```python
from build123d import *

# Parameters (mm, degrees)
BOSS_EXTRUDE1_DEPTH = 700
SKETCH3_W           = 125
SKETCH3_H           = 60
CUT_EXTRUDE1_DEPTH  = 706.00443261
CHAMFER1_SIZE       = 30
SKETCH4_R           = 10
CUT_EXTRUDE2_DEPTH  = 708.990112925
SKETCH5_R           = 7.5
CUT_EXTRUDE3_DEPTH  = 708.990112925
CHAMFER2_SIZE       = 3
FILLET1_R           = 3


with BuildPart() as part:
    # Sketch1 → Boss-Extrude1 (new body)
    with BuildSketch(Plane.XY):
        Polygon((0, -37.5), (0, 37.5), (75, 37.5), (75, 31.15), (6.35, 31.15), (6.35, -31.15), (75, -31.15), (75, -37.5), align=None)
    extrude(amount=BOSS_EXTRUDE1_DEPTH)

    # Sketch3 → Cut-Extrude1 (cut, through all)
    with BuildSketch(Plane.ZY):
        with Locations((92.5, 0)):
            Rectangle(SKETCH3_W, SKETCH3_H)
        with Locations((607.5, 0)):
            Rectangle(SKETCH3_W, SKETCH3_H)
        Polygon((400, 10.383333333), (373, 10.383333333), (373, 31.15), (327, 31.15), (307, 31.15), (307, 10.383333333), (300, 10.383333333), (270, 10.383333333), (270, -10.383333333), (300, -10.383333333), (327, -10.383333333), (327, -31.15), (373, -31.15), (393, -31.15), (393, -10.383333333), (400, -10.383333333), align=None)
    extrude(amount=-CUT_EXTRUDE1_DEPTH, mode=Mode.SUBTRACT)

    # Chamfer1
    chamfer1_edges = [part.edges().sort_by_distance(p)[0] for p in [
        (75, -34.325, 0),
        (75, 34.325, 700),
        (75, -34.325, 700),
        (75, 34.325, 0),
    ]]
    chamfer(chamfer1_edges, length=CHAMFER1_SIZE)

    # Sketch4 → Cut-Extrude2 (cut, through all)
    with BuildSketch(Plane(origin=(0, 37.5, 0), x_dir=(1, 0, 0), z_dir=(0, 1, 0))):
        with Locations(Location((37.5, -607.5, 0), (0, 0, 270))):
            Circle(SKETCH4_R)
        with Locations(Location((37.5, -92.5, 0), (0, 0, 270))):
            Circle(SKETCH4_R)
    extrude(amount=-CUT_EXTRUDE2_DEPTH, mode=Mode.SUBTRACT)

    # Sketch5 → Cut-Extrude3 (cut, through all)
    with BuildSketch(Plane.XZ.offset(37.5)):
        with Locations(Location((38, 273.823015652, 0), (0, 0, 270))):
            Circle(SKETCH5_R)
        with Locations(Location((13.565044391, 350, 0), (0, 0, 270))):
            Circle(SKETCH5_R)
    extrude(amount=-CUT_EXTRUDE3_DEPTH, mode=Mode.SUBTRACT)

    # Chamfer2
    chamfer2_edges = [part.edges().sort_by_distance(p)[0] for p in [
        (6.35, -20.766666667, 327),
        (6.35, 0, 270),
        (6.35, 20.766666667, 373),
        (0, -20.766666667, 393),
        (0, 20.766666667, 307),
    ]]
    chamfer(chamfer2_edges, length=CHAMFER2_SIZE)

    # Fillet1
    fillet1_edges = [part.edges().sort_by_distance(p)[0] for p in [
        (1.675, 10.383333333, 270),
        (1.675, -10.383333333, 270),
        (1.675, 31.15, 373),
        (1.675, -31.15, 327),
        (4.675, -31.15, 393),
        (4.675, 31.15, 307),
        (3.175, 10.383333333, 400),
        (3.175, -10.383333333, 400),
    ]]
    fillet(fillet1_edges, radius=FILLET1_R)


solid = part.part
```
Model file for the job. Use its own axes, mm. A direction names the side the tool comes from. Coordinates: 2 decimals unless noted, no trailing zeros. Order: outer loops, then holes, each group sorted by start corner. A loop starts at its lowest first (then second) coordinate and runs counter-clockwise, first axis right, second up. Notation, with made-up numbers: (-20, 0) - (27, 0) arc R27 ccw to (27, 27) - close; hole circle Ø6 at (86.5, 1). An arc over 180 degrees is marked (long way). Return JSON: item names as keys, results as strings. Group by question number.
1) Saw through at D-D, the plane z = 364. Write the cut outline in (x, y).
2) Tool access for faces 1 (the flat face through (0, -34, 345)), 2 (the flat face through (6.35, 0, 500)): list every direction of +Z, -Z, +X, -X, +Y, -Y with a clear straight run to the whole face (end or side of a thin tool).
3) Saw through at B-B, the plane x = 57.5. Write the cut outline in (y, z).
4) Saw through at A-A, the plane z = 92.5. Write the cut outline in (x, y), plus the area to 3 significant figures.
5) Probe line 1 (Y direction, x = 41.5, z = 585.5); line 2 (X direction, y = -36, z = 92); line 3 (X direction, y = 33, z = 350). List the from-to ranges inside material, lowest first. Write a range as from..to.
6) Flat gauge pin, fed straight in: P1, Ø9, axis at x = 13.57, z = 350, coming from the -Y side. Where does the tip first touch, or does it go through?
7) Mould opens along Z. For faces 3 (the flat face through (60, 34, 685)), 4 (the flat face through (60, 34, 15)), 5 (the cylindrical face through (33.67, -34.281, 616.737)) say: released by +Z, released by -Z, zero draft, split by the parting line, or undercut.
8) Saw through at C-C, the plane y = -1.5. Write the cut outline in (x, z), plus the area to 3 significant figures.
Values found:
{
 "1": {"outline": "(0, -37.5) - (75, -37.5) - (75, -31.15) - (0, -31.15) - close; (0, 31.15) - (75, 31.15) - (75, 37.5) - (0, 37.5) - close"},
 "2": {"face 1": "+Z, -Z, -X, +Y, -Y", "face 2": "+Z, -Z, +X"},
 "3": {"outline": "(-37.5, 12.5) - (-31.15, 12.5) - (-31.15, 687.5) - (-37.5, 687.5) - close; (31.15, 12.5) - (37.5, 12.5) - (37.5, 687.5) - (31.15, 687.5) - close"},
 "4": {"outline": "(0, -37.5) - (27.5, -37.5) - (27.5, -31.15) - (6.35, -31.15) - (6.35, -30) - (0, -30) - close; (0, 30) - (6.35, 30) - (6.35, 31.15) - (27.5, 31.15) - (27.5, 37.5) - (0, 37.5) - close; (47.5, -37.5) - (75, -37.5) - (75, -31.15) - (47.5, -31.15) - close; (47.5, 31.15) - (75, 31.15) - (75, 37.5) - (47.5, 37.5) - close", "area": "713 mm²"},
 "5": {"line 1": "y = -37.5..-31.15, 31.15..37.5", "line 2": "x = 0..27.51, 47.49..75", "line 3": "x = 0..6.07, 21.07..75"},
 "6": {"P1": "passes through"},
 "7": {"face 3": "released by +Z", "face 4": "released by -Z", "face 5": "undercut"},
 "8": {"outline": "(0, 0) - (6.35, 0) - (6.35, 30) - (0, 30) - close; (0, 155) - (6.35, 155) - (6.35, 267) - (3.35, 270) - (0, 270) - close; (0, 400) - (6.35, 400) - (6.35, 545) - (0, 545) - close; (0, 670) - (6.35, 670) - (6.35, 700) - (0, 700) - close", "area": "2,030 mm²"}
}
